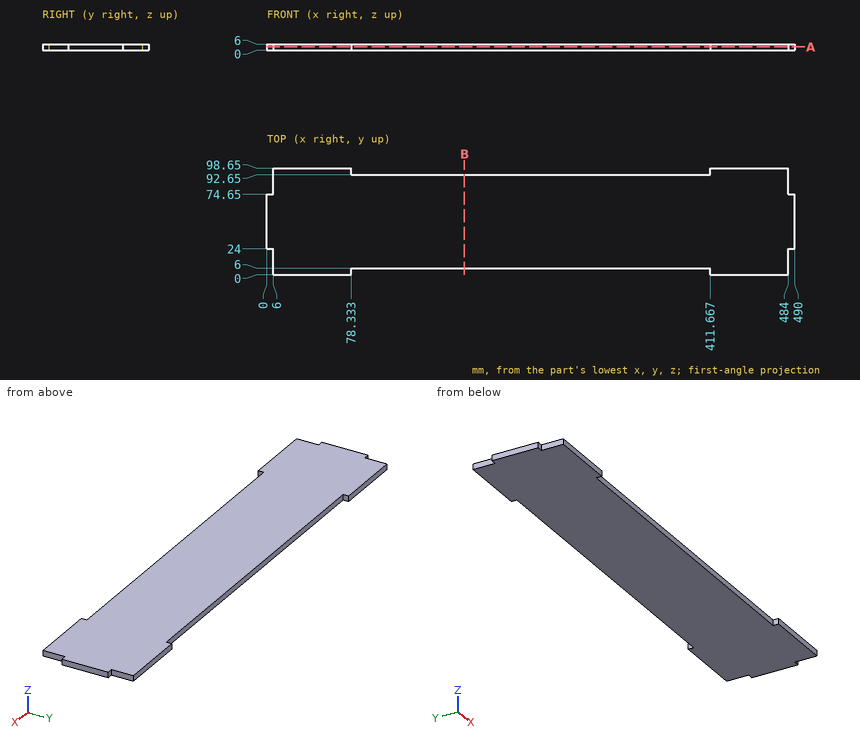
Geometry check sheet. Reference: drawing and pictorial views, mm from the part's lowest x, y, z. Give positions to 0.01 mm unless a question says otherwise; leave off trailing zeros. Loops run counter-clockwise (first coordinate to the right, second up) from the corner with the lowest first, then second, coordinate; pieces in that order, holes last. Notation, with made-up numbers: (13.25, 6) - (37.25, 6) arc R22 ccw to (37.25, 25) - close; hole circle Ø4 at (23.5, -15.5). An arc over 180 degrees is marked (long way). Use CSV: the item, a comma, the result in double quotes. Start each with the question number.
Q1. Go/stop test with flat-tipped pins: pin 1 Ø1.8 at (x, z) = (4.5, 3) entering from -Y; pin 2 Ø3 at (y, z) = (1.5, 4) entering from +X; pin 3 Ø3 at (x, z) = (104.5, 5) entering from +Y. Record where each tip stops, or that it passes through.
Q2. Section check B-B, the plane x = 183.5. Record the cut outline in (y, z).
Q3. Section check A-A, the plane z = 3.25. Record the cut outline in (x, y).
Q4. Scan lines: probe 1 along X at (y, z) = (14, 5.75); probe 2 along Y at (x, z) = (87, 4). Record each from-to range of solid material in increasing order. Write a range as from..to.
Findings below:
1,pin 1,"stops at y = 24"
1,pin 2,"stops at x = 484"
1,pin 3,"stops at y = 92.65"
2,outline,"(6, 0) - (92.65, 0) - (92.65, 6) - (6, 6) - close"
3,outline,"(0, 24) - (6, 24) - (6, 0) - (78.33, 0) - (78.33, 6) - (411.67, 6) - (411.67, 0) - (484, 0) - (484, 24) - (490, 24) - (490, 74.65) - (484, 74.65) - (484, 98.65) - (411.67, 98.65) - (411.67, 92.65) - (78.33, 92.65) - (78.33, 98.65) - (6, 98.65) - (6, 74.65) - (0, 74.65) - close"
4,probe 1,"x = 6..484"
4,probe 2,"y = 6..92.65"
